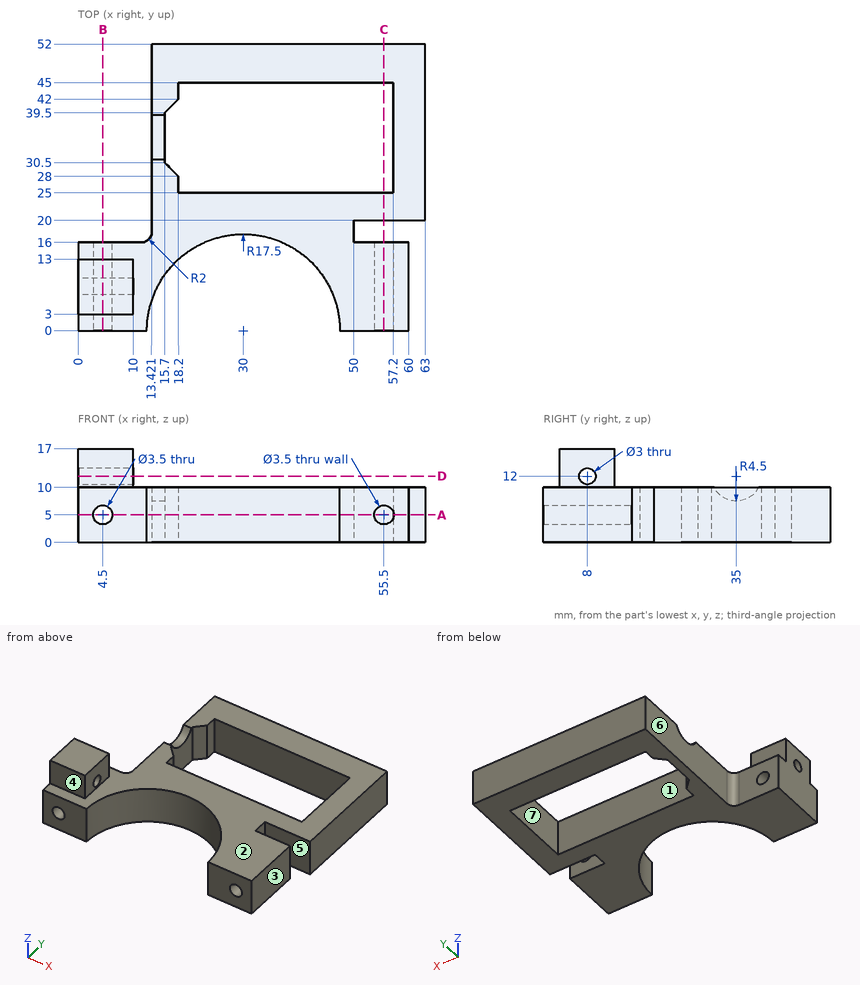
Answer from the drawing. Dimensions are ordinates in mm from the lowest x, y and z of the part. A direction names the side the tool comes from. Round coordinates to 2 decimals unless told otherwise and drop trailing zeros. Order: outer loops, then holes, each group sorted by start corner. A loop starts at its lowest first (then second) coordinate and runs counter-clockwise, first axis right, second up. Notation, with made-up numbers: (60.25, -1.5) -> (110.25, -1.5) arc R17 ccw to (110.25, 15.5) -> close; hole circle Ø1 at (-17.75, 50). An arc over 180 degrees is marked (long way). Answer as CSV lines item,"result".
Q1. Which of the six approach directions +Z, -Z, +X, -X, +Y, -Y give full straight-line access (tool end or side, diameter ignored) to the marked faces 4, 5, 6 and 7?
Computed values:
face 4,"+Z, +X, -X, -Y"
face 5,"+Z, -Z, +X"
face 6,"+Z, -Z, -X, +Y"
face 7,"+Z, -Z"
Q2. A cutting plane is placed at A-A on z = 5. Give the number of separate pieces and of enclosed holes in the cut face, plus the area to 3 significant figures.
Computed values:
separate pieces,"3"
enclosed holes,"1"
area,"1,290 mm^2"
Q3. A cutting plane is placed at B-B on x = 4.5. Determine the outline of the cut face in (y, z).
Computed values:
outline,"(0, 0) -> (16, 0) -> (16, 3.25) -> (0, 3.25) -> close; (0, 6.75) -> (16, 6.75) -> (16, 10) -> (13, 10) -> (13, 17) -> (3, 17) -> (3, 10) -> (0, 10) -> close; hole circle Ø3 at (8, 12)"
Q4. For a pull along X with two mould halves and no side action, classify the marked faces 1, 2 and 3 as +X half, -X half, draft (parallel to the pull), parting line (faces both ways), or undercut.
Computed values:
face 1,"undercut"
face 2,"draft"
face 3,"+X half"
Q5. A cutting plane is placed at D-D on z = 12. Determine the outline of the cut face in (x, y).
Computed values:
outline,"(0, 3) -> (10, 3) -> (10, 6.5) -> (0, 6.5) -> close; (0, 9.5) -> (10, 9.5) -> (10, 13) -> (0, 13) -> close"
Q6. Given pin 1 (8 mm diameter, centred on y = 11.5, z = 2.5, fed in from +X); pin 2 (3 mm diameter, centred on y = 32, z = 3, fed in from -X); pin 3 (8 mm diameter, centred on x = 7, z = 5.5, fed in from +Y), each flat-ended and moving along its own axis, determine where each tip first touches the part or whether it passes through.
Computed values:
pin 1,"stops at x = 60"
pin 2,"stops at x = 13.42"
pin 3,"stops at y = 16"
Q7. A cutting plane is placed at C-C on x = 55.5. Determine the outline of the cut face in (y, z), plus the area to 3 significant figures.
Computed values:
outline,"(0, 0) -> (16, 0) -> (16, 3.25) -> (0, 3.25) -> close; (0, 6.75) -> (16, 6.75) -> (16, 10) -> (0, 10) -> close; (20, 0) -> (25, 0) -> (25, 10) -> (20, 10) -> close; (45, 0) -> (52, 0) -> (52, 10) -> (45, 10) -> close"
area,"224 mm^2"
Q8. Consider line 1 (Z direction, x = 4.5, y = 5); line 2 (X direction, y = 33, z = 3); line 3 (Z direction, x = 55.5, y = 7.75). Determine where each line is inside the solid, lowest interval first. Write a range as from..to.
Computed values:
line 1,"z = 0..3.25, 6.75..17"
line 2,"x = 13.42..15.7, 57.2..63"
line 3,"z = 0..3.25, 6.75..10"
